from build123d import *

# Parameters (mm, degrees)
SKETCH1_W           = 170
SKETCH1_H           = 170
BOSS_EXTRUDE1_DEPTH = 100
FILLET1_R           = 50


with BuildPart() as part:
    # Sketch1 → Boss-Extrude1 (new body)
    with BuildSketch(Plane.XY):
        with Locations((85, 85)):
            Rectangle(SKETCH1_W, SKETCH1_H)
    extrude(amount=BOSS_EXTRUDE1_DEPTH)

    # Fillet1
    fillet1_edges = [part.edges().sort_by_distance(p)[0] for p in [
        (85, 0, 0),
        (170, 85, 0),
        (85, 170, 0),
        (0, 85, 0),
        (85, 170, 100),
        (170, 85, 100),
        (85, 0, 100),
        (0, 85, 100),
    ]]
    fillet(fillet1_edges, radius=FILLET1_R - 0.0001)  # a hair under: the kernel refuses the full size


solid = part.part
Here's how the part is built. I have some questions about the finished solid (model axes, mm). Round coordinates to 2 decimals unless told otherwise and drop trailing zeros. Loops run counter-clockwise (first coordinate to the right, second up) from the corner with the lowest first, then second, coordinate; pieces in that order, holes last. Notation, with made-up numbers: M -25,-39 L 0,-39 A20 ccw 0,-25 Z; hole C 41.25,12.25 d4. An arc over 180 degrees is marked long. Write each question's results on one line, items separated by ' | '. Start each with the question number.
(1) If I drill on probe 1 along Y at (x, z) = (45, 49.5); probe 2 along Y at (x, z) = (10.5, 40.5), over which ranges is the centre line in solid material (lowest first)? Write a range as from..to.
(2) I want a section at D-D (z = 89). Please give me the cut outline in (x, y), then the cut area to 3 significant figures.
(3) I want a section at C-C (z = 41.5). Please give me the cut outline in (x, y).
(4) Will these pins go through, and if not, where does the flat tip stop? P1, Ø12, axis at x = 134, z = 72.5, coming from the -Y side; P2, Ø2, axis at x = 111, y = 47, coming from the +Z side; P3, Ø5, axis at x = 117.5, y = 43.5, coming from the -Z side.
Solved:
1) probe 1: y = 0..170 | probe 2: y = 0.91..169.09
2) outline: M 18.71,18.71 L 151.29,18.71 L 151.29,151.29 L 18.71,151.29 Z | area: 17,600 mm²
3) outline: M 0.73,0.73 L 169.27,0.73 L 169.27,169.27 L 0.73,169.27 Z
4) P1: stops at y = 2.8 | P2: stops at z = 99.96 | P3: stops at z = 0.16
